CAD build for the part. Positions are in the model's coordinates, mm. A direction names the side the tool comes from. Round coordinates to 2 decimals unless told otherwise and drop trailing zeros. Loops run counter-clockwise (first coordinate to the right, second up) from the corner with the lowest first, then second, coordinate; pieces in that order, holes last. Notation, with made-up numbers: M 44.25,-36.5 L 54.25,-36.5 A18 cw 54.25,-1.5 Z; hole C 89.25,-21.75 d5. An arc over 180 degrees is marked long. Use one line per item in the form item = value.
from build123d import *

# Parameters (mm, degrees)
F0_R     = 8.9668874309
F1_DEPTH = 19.05
F2_R     = 8.9668874309
F3_DEPTH = 76.2
F4_R     = 9.2392486584
F5_DEPTH = 19.05
F6_DEPTH = 19.05


with BuildPart() as f1:
    # F0 (on Front) → F1 (new body)
    with BuildSketch(Plane.XZ):
        with BuildLine():
            Line((-23.8205983585, 48.6063640565), (-23.8205983585, -30.8263637125))
            ThreePointArc((-23.8205983585, -30.8263637125), (0, -54.6469620711), (23.8205983585, -30.8263637125))
            Line((23.8205983585, -30.8263637125), (23.8205983585, 48.6063640565))
            ThreePointArc((23.8205983585, 48.6063640565), (0, 72.426962415), (-23.8205983585, 48.6063640565))
        make_face()
        with Locations((0, -30.8263637125)):
            Circle(F0_R, mode=Mode.SUBTRACT)
        with Locations((0.2309088741, 48.3754538)):
            Circle(F0_R, mode=Mode.SUBTRACT)
    extrude(amount=F1_DEPTH)

    # F2 (on face) → F3 (join)
    with BuildSketch(Plane.XZ.offset(19.05)):
        with BuildLine():
            ThreePointArc((-23.8205983585, -30.8263637125), (0, -54.6469620711), (23.8205983585, -30.8263637125))
            ThreePointArc((23.8205983585, -30.8263637125), (0, -7.005765354), (-23.8205983585, -30.8263637125))
        make_face()
        with Locations((0, -30.8263637125)):
            Circle(F2_R, mode=Mode.SUBTRACT)
    extrude(amount=F3_DEPTH)

    # F4 (on face) → F5 (join)
    with BuildSketch(Plane.XZ.offset(95.25)):
        with BuildLine():
            Line((-23.8205983585, 45.3295558312), (-23.8205983585, -29.759446989))
            ThreePointArc((-23.8205983585, -29.759446989), (-0.5335919833, -54.6648724127), (23.8444798109, -30.8263637125))
            Line((23.8444798109, -30.8263637125), (24.0145456046, -30.8263637125))
            Line((24.0145456046, -30.8263637125), (24.0145456046, 48.3754538))
            ThreePointArc((24.0145456046, 48.3754538), (-1.5260332541, 72.3414635451), (-23.8205983585, 45.3295558312))
        make_face()
        with BuildLine():
            ThreePointArc((23.8205983585, -30.8263637125), (0, -54.6469620711), (-23.8205983585, -30.8263637125))
            ThreePointArc((-23.8205983585, -30.8263637125), (0, -7.005765354), (23.8205983585, -30.8263637125))
        make_face(mode=Mode.SUBTRACT)
        with Locations((0, 48.3754538)):
            Circle(F4_R, mode=Mode.SUBTRACT)
    extrude(amount=F5_DEPTH)

    # F6 (add): a face of the model
    f6_faces = [f1.faces().sort_by_distance(p)[0] for p in [
        (-23.1468500933, -95.25, -30.8263637125),
    ]]
    extrude(f6_faces, amount=F6_DEPTH)


solid = f1.part
1. Tool access for faces 1 (the face through (23.821, -9, 8)), 2 (the face through (24.015, -105, 8)): list every direction of +Z, -Z, +X, -X, +Y, -Y with a clear straight run to the whole face (end or side of a thin tool).
Completed:
face_1 = +Z, -Z, +X, +Y
face_2 = +Z, -Z, +X, +Y, -Y
2. Cut at C-C on z = 43.5. Write the cut outline in (x, y).
Completed:
outline = M -23.82,-114.3 L -7.85,-114.3 L -7.85,-95.25 L -23.82,-95.25 Z; M -23.82,-19.05 L -7.29,-19.05 L -7.29,0 L -23.82,0 Z; M 7.76,-19.05 L 23.82,-19.05 L 23.82,0 L 7.76,0 Z; M 7.85,-114.3 L 24.01,-114.3 L 24.01,-95.25 L 7.85,-95.25 Z
3. Drop flat-ended pins along their axis: P1, Ø3, axis at x = 11.5, y = -48.5, coming from the +Z side; P2, Ø21, axis at y = -7.5, z = -7.5, coming from the -X side; P3, Ø3, axis at x = 18.5, y = -43.5, coming from the -Z side. Give the stop position or say it passes through.
Completed:
P1 = -9.21
P2 = -23.82
P3 = -47.51
4. Cut at B-B on y = -9.5. Write the cut outline in (x, z), and give its area (3 significant figures).
Completed:
outline = M -23.82,-30.83 A23.82 ccw 23.82,-30.83 L 23.82,48.61 A23.82 ccw -23.82,48.61 Z; hole C 0,-30.83 d17.93; hole C 0.23,48.38 d17.93
area = 5,060 mm2
5. Cut at A-A on z = 29.5. Write the cut outline in (x, y), and give its area (3 significant figures).
Completed:
outline = M -23.82,-114.3 L 24.01,-114.3 L 24.01,-95.25 L -23.82,-95.25 Z; M -23.82,-19.05 L 23.82,-19.05 L 23.82,0 L -23.82,0 Z
area = 1,820 mm2
6. Cut at D-D on x = 0. State how many separate pieces and enclosed holes the cut face has, and give its area (3 significant figures).
Completed:
separate_pieces = 4
enclosed_holes = 0
area = 5,730 mm2
7. Pull direction Z, two halves, no side cores. Call faces 3 (the face through (-1.203, -104.642, 57.536)), 4 (the face through (-23.821, -9, 9)), 5 (the face through (0.52, -9.39, 72.42)): +Z half, -Z half, draft (parallel to the pull), parting line (faces both ways), or undercut.
Completed:
face_3 = undercut
face_4 = draft
face_5 = +Z half
8. Probe line 1 along Z through (x, y) = (0, -103); line 2 along Y through (x, z) = (22, 38); line 3 along Z through (x, y) = (0, -70.5). List the from-to ranges inside material, lowest first. Write a range as from..to.
Completed:
line_1 = -54.67..-39.79, -21.86..39.14, 57.61..72.39
line_2 = -114.3..-95.25, -19.05..0
line_3 = -54.65..-39.79, -21.86..-7.01
